Check sheet for the modelled part. Datum: model origin and axes. Units: mm. A direction names the side the tool comes from. Round coordinates to 2 decimals unless told otherwise and drop trailing zeros. Loops run counter-clockwise (first coordinate to the right, second up) from the corner with the lowest first, then second, coordinate; pieces in that order, holes last. Notation, with made-up numbers: (1.25, 51) - (55.25, 51) arc R37 cw to (55.25, 89) - close; hole circle Ø9 at (14, 52.25). An arc over 180 degrees is marked (long way). Put each result on its own line as item: value. Start each with the question number.
Item 1: Draft check along Y on faces 3 (the flat face through (-8, 6.9, 0)), 4 (the flat face through (-6, 4.5, 0)), 5 (the cylindrical face through (-9.5, 6.11, -0.07)). Enter one of: pulls with the +Y half, pulls with the -Y half, needs draft (parallel to the pull), parting line crosses it, or undercut.
Item 2: Section check C-C, the plane y = 5.5. Record the cut outline in (x, z).
Item 3: Tool access check on faces 1 (the flat face through (-6, 5.3, 0)), 2 (the cylindrical face through (-5.56, 4.91, 0.54)). Record the directions out of +Z, -Z, +X, -X, +Y, -Y that give a thin tool (end or side, any length) a straight path to the whole face; none if there is none.
Item 4: Section check D-D, the plane z = 0. Record the cut outline in (x, y).
Item 5: Section check B-B, the plane z = 1.8. Record the cut outline in (x, y).
Item 6: Gauge pin test, flat end, axial feed: pin 1 Ø1.5 at (x, z) = (-9, 0.5) entering from -Y. Record the tip position at first contact, or that the pin passes through.
Item 7: Material ranges on line 1 along Y through (x, z) = (-9.3, 1.5); line 2 along Z through (x, y) = (-8.05, 5.75); line 3 along Y through (x, z) = (-9.9, 0.8), recorded low to high.
Item 8: Section check A-A, the plane x = -8. Record the cut outline in (y, z), and give its area (3 significant figures).
from build123d import *

# Parameters (mm, degrees)
SKETCH1_W                = 2.5
SKETCH1_H                = 0.8
SURFACE_EXTRUDE1_1_BACK  = 5
SURFACE_EXTRUDE1_1_DEPTH = 10


# Read off the part's stored shape, not the designer's step: Stock-Ball_socket_test-1
with BuildPart() as part:
    # Stock-Ball_socket_test-1 outline → Stock-Ball_socket_test-1 (revolve)
    with BuildSketch(Plane(origin=(-8, 0, 0), x_dir=(1, 0, 0), z_dir=(0, 0, 1))):
        with BuildLine():
            ThreePointArc((0, 0), (1.767766953, 0.732233047), (2.5, 2.5))
            ThreePointArc((2.5, 2.5), (2.236067977, 3.618033989), (1.5, 4.5))
            Line((1.5, 4.5), (1.5, 7.5))
            Line((1.5, 7.5), (0, 7.5))
            Line((0, 7.5), (0, 0))
        make_face()
    revolve(axis=Axis((-8, 0, 0), (0, 1, 0)))

    # Sketch1 → Revolve1 (revolve)
    with BuildSketch(Plane.XY, mode=Mode.PRIVATE) as revolve1_sk:
        with Locations((-9.25, 4.9)):
            Rectangle(SKETCH1_W, SKETCH1_H)
    revolve(revolve1_sk.sketch.rotate(Axis((-8, 0, 0), (0, 1, 0)), 270), axis=Axis((-8, 0, 0), (0, 1, 0)))

    # SurfaceCut1: cut with a surface, the side behind it stays
    # Surface-Extrude1: a surface, the sketch's curves swept straight by 10 mm
    with BuildLine(Plane.XY.offset(-SURFACE_EXTRUDE1_1_BACK), mode=Mode.PRIVATE) as surface_extrude1_1_path:
        Line((-10.166377041, 6.9), (-4.598288461, 6.9))
    surface_extrude1_1 = Shell.extrude(surface_extrude1_1_path.wire(), (0 * SURFACE_EXTRUDE1_1_DEPTH, 0 * SURFACE_EXTRUDE1_1_DEPTH, 1 * SURFACE_EXTRUDE1_1_DEPTH))
    split(bisect_by=surface_extrude1_1, keep=Keep.BOTTOM)


solid = part.part
Check result:
1. face 3: pulls with the +Y half
1. face 4: undercut
1. face 5: needs draft
2. outline: circle Ø3 at (-8, 0)
3. face 1: +Y
3. face 2: +Y, -Y
4. outline: (-10.5, 4.5) - (-9.5, 4.5) arc R2.5 ccw (long way) to (-6.5, 4.5) - (-5.5, 4.5) - (-5.5, 5.3) - (-6.5, 5.3) - (-6.5, 6.9) - (-9.5, 6.9) - (-9.5, 5.3) - (-10.5, 5.3) - close
5. outline: circle Ø3.47 at (-8, 2.5); (-9.73, 4.5) - (-6.27, 4.5) - (-6.27, 5.3) - (-9.73, 5.3) - close
6. pin 1: y = 0.03
7. line 1: 0.98 to 4.02, 4.5 to 5.3
7. line 2: -1.5 to 1.5
7. line 3: 1.09 to 3.91, 4.5 to 5.3
8. outline: (4.5, -2.5) - (5.3, -2.5) - (5.3, -1.5) - (6.9, -1.5) - (6.9, 1.5) - (5.3, 1.5) - (5.3, 2.5) - (4.5, 2.5) - (4.5, 1.5) arc R2.5 ccw (long way) to (4.5, -1.5) - close
8. area: 27.4 mm²
